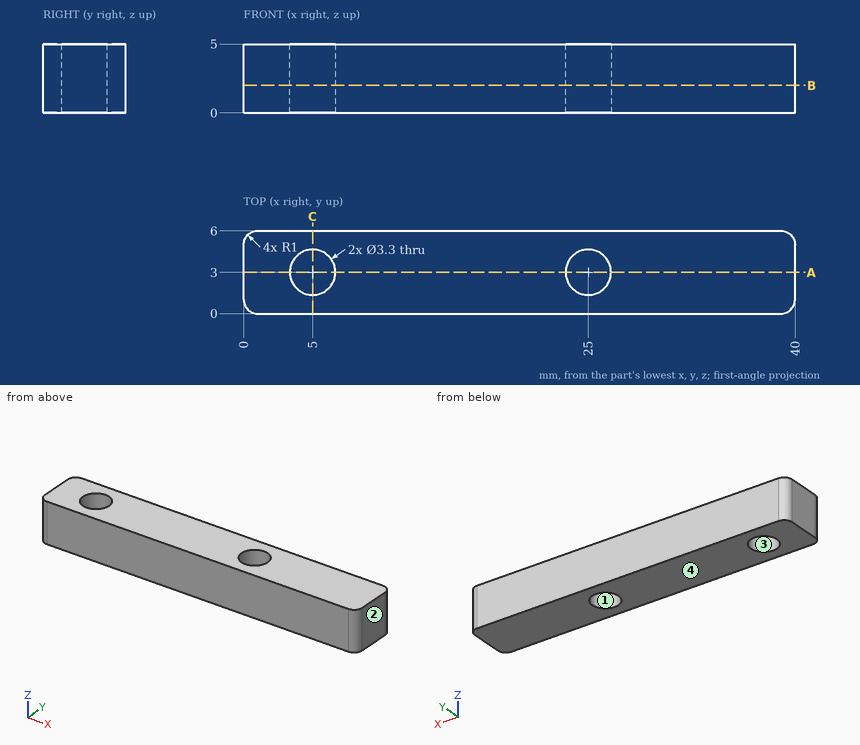
Print and shaded views of the part. All mm, measured from the part's lowest x, y and z. Coordinates: 2 decimals unless noted, no trailing zeros. Order: outer loops, then holes, each group sorted by start corner. A loop starts at its lowest first (then second) coordinate and runs counter-clockwise, first axis right, second up. Notation, with made-up numbers: (-32.5, -14.5) - (-27.5, -14.5) arc R19 ccw to (-27.5, -4.5) - close; hole circle Ø1 at (-5.5, 38.25). An arc over 180 degrees is marked (long way). Return JSON: item names as keys, results as strings. Group by question number.
Item 1: Cut at C-C (x = 5). List the corners of the cut face in (y, z), plus the area to 3 significant figures.
Item 2: Pull direction X, two halves, no side cores. Call the marked faces 1, 2, 3 and 4: pulls with the +X half, pulls with the -X half, needs draft (parallel to the pull), parting line crosses it, or undercut.
Item 3: Cut at B-B (z = 2). List the corners of the cut face in (x, y).
Item 4: Drill centre lines: probe 1 along X at (y, z) = (4.4, 0.4); probe 2 along Y at (x, z) = (25, 2.4); probe 3 along X at (y, z) = (4.25, 2.75). Where is each one in solid material? Low to high. Write a range as from..to.
Item 5: Cut at A-A (y = 3). List the corners of the cut face in (x, z).
Check values:
{
 "1": {"outline": "(0, 0) - (1.35, 0) - (1.35, 5) - (0, 5) - close; (4.65, 0) - (6, 0) - (6, 5) - (4.65, 5) - close", "area": "13.5 mm2"},
 "2": {"face 1": "undercut", "face 2": "pulls with the +X half", "face 3": "undercut", "face 4": "needs draft"},
 "3": {"outline": "(0, 1) arc R1 ccw to (1, 0) - (39, 0) arc R1 ccw to (40, 1) - (40, 5) arc R1 ccw to (39, 6) - (1, 6) arc R1 ccw to (0, 5) - close; hole circle Ø3.3 at (5, 3); hole circle Ø3.3 at (25, 3)"},
 "4": {"probe 1": "x = 0..4.13, 5.87..24.13, 25.87..40", "probe 2": "y = 0..1.35, 4.65..6", "probe 3": "x = 0..3.92, 6.08..23.92, 26.08..40"},
 "5": {"outline": "(0, 0) - (3.35, 0) - (3.35, 5) - (0, 5) - close; (6.65, 0) - (23.35, 0) - (23.35, 5) - (6.65, 5) - close; (26.65, 0) - (40, 0) - (40, 5) - (26.65, 5) - close"}
}
